Part print with two shaded views. Sizes in mm from the minimum x, y, z corner. A direction names the side the tool comes from. Give positions to 0.01 mm unless a question says otherwise; leave off trailing zeros. Order: outer loops, then holes, each group sorted by start corner. A loop starts at its lowest first (then second) coordinate and runs counter-clockwise, first axis right, second up.
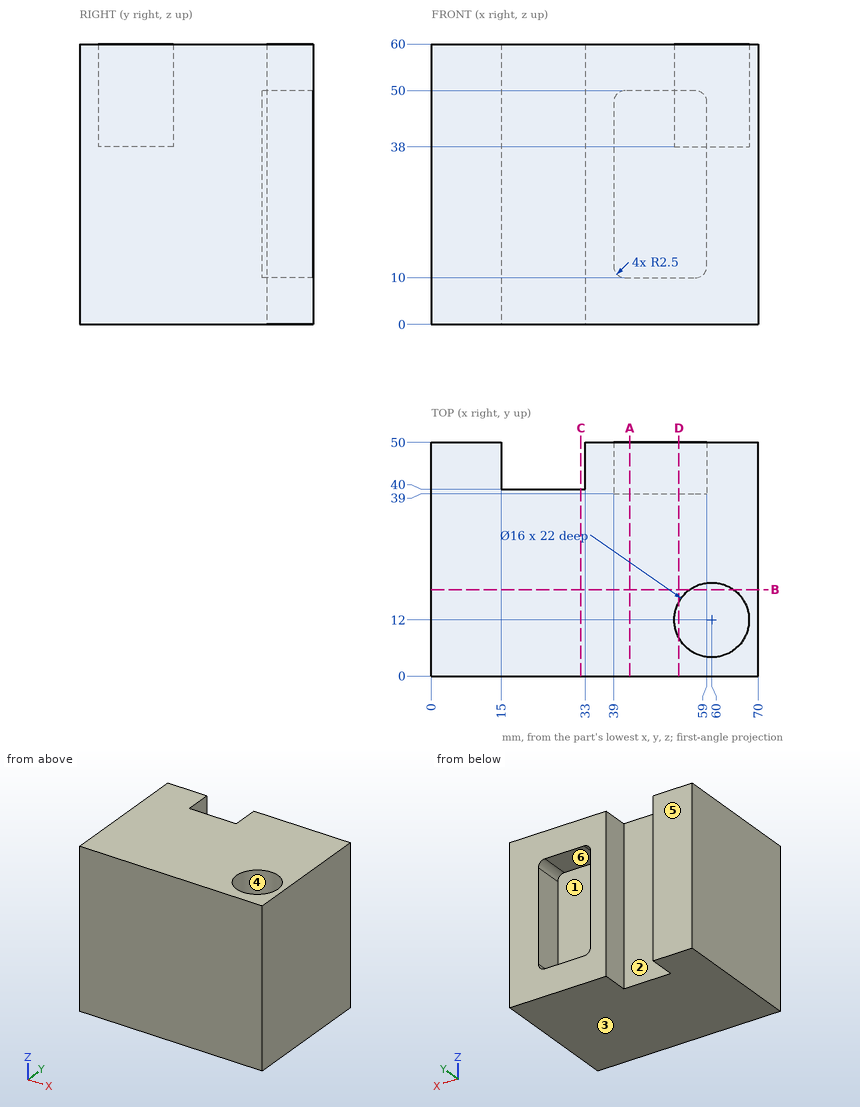
Item 1: Slice it at D-D (x = 53). Give the cut face in (y, z), and give its area (3 significant figures).
Item 2: Two-plate mould, pull along Y, no slides. Class the marked faces 4, 5 and 6: released by +Y, released by -Y, zero draft, split by the parting line, or undercut.
Item 3: Slice it at B-B (y = 18.5). Give the cut face in (x, z), and give its area (3 significant figures).
Item 4: Wall check: L1, parallel to X at y = 44, z = 27.5; L2, parallel to Y at x = 60, z = 51; L3, parallel to Z at x = 53, y = 43. Give the ranges that are in metal, low to high.
Item 5: Tool access for the marked faces 1, 2 and 3: list every direction of +Z, -Z, +X, -X, +Y, -Y with a clear straight run to the whole face (end or side of a thin tool).
Item 6: Drop flat-ended pins along their axis: pin 1 Ø6 at (x, z) = (45.5, 26) entering from +Y; pin 2 Ø9 at (x, y) = (50, 46) entering from -Z; pin 3 Ø9 at (x, z) = (24.5, 33.5) entering from +Y. Give the stop position or say it passes through.
Item 7: Slice it at C-C (x = 32). Give the cut face in (y, z), and give its area (3 significant figures).
Item 8: Slice it at A-A (x = 42.5). Give the cut face in (y, z).
A:
1. outline: (0, 0) - (50, 0) - (50, 10) - (39, 10) - (39, 50) - (50, 50) - (50, 60) - (15.87, 60) - (15.87, 38) - (8.13, 38) - (8.13, 60) - (0, 60) - close
1. area: 2,390 mm2
2. face 4: undercut
2. face 5: released by +Y
2. face 6: zero draft
3. outline: (0, 0) - (70, 0) - (70, 60) - (64.66, 60) - (64.66, 38) - (55.34, 38) - (55.34, 60) - (0, 60) - close
3. area: 3,990 mm2
4. L1: x = 0 to 15, 33 to 39, 59 to 70
4. L2: y = 0 to 4, 20 to 50
4. L3: z = 0 to 10, 50 to 60
5. face 1: +Y
5. face 2: +Z, -Z, +Y
5. face 3: -Z, +X, -X, +Y, -Y
6. pin 1: stops at y = 39
6. pin 2: stops at z = 0
6. pin 3: stops at y = 40
7. outline: (0, 0) - (40, 0) - (40, 60) - (0, 60) - close
7. area: 2,400 mm2
8. outline: (0, 0) - (50, 0) - (50, 10) - (39, 10) - (39, 50) - (50, 50) - (50, 60) - (0, 60) - close
